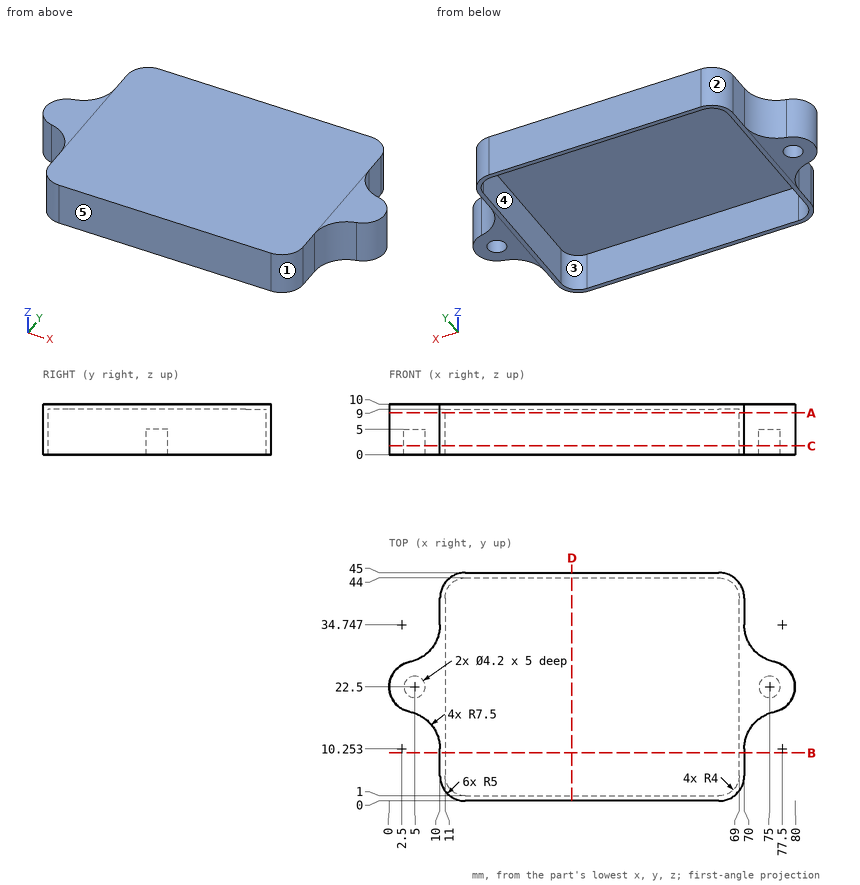
Job drawing, mm, ordinate dimensions from the low corner. One solid piece. A direction names the side the tool comes from. Round coordinates to 2 decimals unless told otherwise and drop trailing zeros. Write each loop counter-clockwise with the first axis right and the second up, starting at its lowest first coordinate (ties: lowest second). Pieces come first, ordered by that corner, then holes.
1) 3-axis set-ups, long thin cutter, end or side, ignore diameter. For the marked faces 4 and 5: which of +Z, -Z, +X, -X, +Y, -Y reach the whole face in a straight line?
2) Band-saw the part on B-B, the plane y = 9.5. List the corners of the cut face in (x, z).
3) Mould opens along X. For the marked faces 1, 2 and 3 say: +X half, -X half, draft (parallel to the pull), parting line (faces both ways), or undercut.
4) Drill centre lines: probe 1 along X at (y, z) = (22.5, 1.45); probe 2 along X at (y, z) = (10.5, 7.5); probe 3 along Y at (x, z) = (25, 7.75). Where is each one in solid material? Low to high.
5) Pin check, flat tips, straight feed: pin 1 (2.5 mm diameter, centred on y = 8.5, z = 4.5, fed in from -X); pin 2 (1 mm diameter, centred on y = 21.5, z = 6, fed in from +X) (1 decimal); pin 3 (8 mm diameter, centred on x = 42, y = 29, fed in from -Z); pin 4 (6.5 mm diameter, centred on x = 5, y = 22.5, fed in from -Z). Stop position of each tip, or through.
6) Band-saw the part on C-C, the plane z = 1.75. List the corners of the cut face in (x, y).
7) Band-saw the part on D-D, the plane x = 36. List the corners of the cut face in (y, z).
8) Band-saw the part on A-A, the plane z = 8.25. List the corners of the cut face in (x, y), and give its area (3 significant figures).
Ans:
1. face 4: -Z
1. face 5: +Z, -Z, +X, -X, -Y
2. outline: (10, 0) - (11, 0) - (11, 9) - (69, 9) - (69, 0) - (70, 0) - (70, 10) - (10, 10) - close
3. face 1: +X half
3. face 2: -X half
3. face 3: undercut
4. probe 1: x = 0 to 2.9, 7.1 to 11, 69 to 72.9, 77.1 to 80
4. probe 2: x = 10 to 11, 69 to 70
4. probe 3: y = 0 to 1, 44 to 45
5. pin 1: stops at x = 10
5. pin 2: stops at x = 80
5. pin 3: stops at z = 9
5. pin 4: stops at z = 0
6. outline: (4, 17.6) arc R7.5 cw to (10, 10.25) - (10, 5) arc R5 ccw to (15, 0) - (65, 0) arc R5 ccw to (70, 5) - (70, 10.25) arc R7.5 cw to (76, 17.6) arc R5 ccw to (76, 27.4) arc R7.5 cw to (70, 34.75) - (70, 40) arc R5 ccw to (65, 45) - (15, 45) arc R5 ccw to (10, 40) - (10, 34.75) arc R7.5 cw to (4, 27.4) arc R5 ccw to start; hole circle Ø4.2 at (5, 22.5); hole (11, 5) arc R4 ccw to (15, 1) - (65, 1) arc R4 ccw to (69, 5) - (69, 40) arc R4 ccw to (65, 44) - (15, 44) arc R4 ccw to (11, 40) - close; hole circle Ø4.2 at (75, 22.5)
7. outline: (0, 0) - (1, 0) - (1, 9) - (44, 9) - (44, 0) - (45, 0) - (45, 10) - (0, 10) - close
8. outline: (4, 17.6) arc R7.5 cw to (10, 10.25) - (10, 5) arc R5 ccw to (15, 0) - (65, 0) arc R5 ccw to (70, 5) - (70, 10.25) arc R7.5 cw to (76, 17.6) arc R5 ccw to (76, 27.4) arc R7.5 cw to (70, 34.75) - (70, 40) arc R5 ccw to (65, 45) - (15, 45) arc R5 ccw to (10, 40) - (10, 34.75) arc R7.5 cw to (4, 27.4) arc R5 ccw to start; hole (11, 5) arc R4 ccw to (15, 1) - (65, 1) arc R4 ccw to (69, 5) - (69, 40) arc R4 ccw to (65, 44) - (15, 44) arc R4 ccw to (11, 40) - close
8. area: 419 mm2
